Input: part model. Units: mm. Frame: model coordinates. Coordinates: 2 decimals unless noted, no trailing zeros. Loops run counter-clockwise (first coordinate to the right, second up) from the corner with the lowest first, then second, coordinate; pieces in that order, holes last. Notation, with made-up numbers: (0, 44.25) -> (16, 44.25) arc R18 cw to (16, 54.25) -> close; hole circle Ø3 at (-4, -6.75). An arc over 180 degrees is marked (long way). Answer as a JSON object with one key per item and string values.
from build123d import *

# Parameters (mm, degrees)
SKETCH1_W                  = 76.2
SKETCH1_H                  = 76.2
SKETCH1_R                  = 14.2875
SKETCH1_R_2                = 2.54
INITIAL_PLATE_DEPTH        = 6.35
MOUNTING_PATTERN_OUTLINE_R = 2.54
MOUNTING_PATTERN_DEPTH     = 6.35


# Read off the part's stored shape, not the designer's step: Mounting Pattern
with BuildPart() as part:
    # Sketch1 → Initial Plate (new body)
    with BuildSketch(Plane(origin=(0, 0, 0), x_dir=(1, 0, 0), z_dir=(0, 1, 0))):
        Rectangle(SKETCH1_W, SKETCH1_H)
        with Locations(Location((0, 0, 0), (0, 0, 270))):
            Circle(SKETCH1_R, mode=Mode.SUBTRACT)
        with Locations(Location((-25.4, 0, 0), (0, 0, 270))):
            Circle(SKETCH1_R_2, mode=Mode.SUBTRACT)
    extrude(amount=INITIAL_PLATE_DEPTH)

    # Mounting Pattern outline → Mounting Pattern (cut)
    with BuildSketch(Plane(origin=(0, 0, 0), x_dir=(1, 0, 0), z_dir=(0, 1, 0))):
        with Locations((0, 25.4)):
            Circle(MOUNTING_PATTERN_OUTLINE_R)
        with Locations((25.4, 0)):
            Circle(MOUNTING_PATTERN_OUTLINE_R)
        with Locations((0, -25.4)):
            Circle(MOUNTING_PATTERN_OUTLINE_R)
    extrude(amount=MOUNTING_PATTERN_DEPTH, mode=Mode.SUBTRACT)


solid = part.part
1. Section query A-A (x = 25.4). Return loops of the section in (y, z).
Reply:
{"outline": "(0, -38.1) -> (6.35, -38.1) -> (6.35, -2.54) -> (0, -2.54) -> close; (0, 2.54) -> (6.35, 2.54) -> (6.35, 38.1) -> (0, 38.1) -> close"}
2. Section query C-C (y = 5). Return loops of the section in (x, z) (1 decimal), plus the area to 3 significant figures.
Reply:
{"outline": "(-38.1, -38.1) -> (38.1, -38.1) -> (38.1, 38.1) -> (-38.1, 38.1) -> close; hole circle Ø5.1 at (-25.4, 0); hole circle Ø28.6 at (0, 0); hole circle Ø5.1 at (0, -25.4); hole circle Ø5.1 at (0, 25.4); hole circle Ø5.1 at (25.4, 0)", "area": "5,080 mm2"}
3. Mould query, pull axis Z, two halves, no side actions, for faces 1 (the face through (16, 0, -1)), 2 (the face through (-27.653, 3.131, 1.172)), 3 (the face through (-1, 3, 38.1)). Classes: pulls with the +Z half, pulls with the -Z half, needs draft (parallel to the pull), parting line crosses it, or undercut.
Reply:
{"face 1": "needs draft", "face 2": "undercut", "face 3": "pulls with the +Z half"}
4. Section query B-B (z = 25.4). Return loops of the section in (x, y).
Reply:
{"outline": "(-38.1, 0) -> (-2.54, 0) -> (-2.54, 6.35) -> (-38.1, 6.35) -> close; (2.54, 0) -> (38.1, 0) -> (38.1, 6.35) -> (2.54, 6.35) -> close"}
5. Section query D-D (z = 0). Return loops of the section in (x, y), plus the area to 3 significant figures.
Reply:
{"outline": "(-38.1, 0) -> (-27.94, 0) -> (-27.94, 6.35) -> (-38.1, 6.35) -> close; (-22.86, 0) -> (-14.29, 0) -> (-14.29, 6.35) -> (-22.86, 6.35) -> close; (14.29, 0) -> (22.86, 0) -> (22.86, 6.35) -> (14.29, 6.35) -> close; (27.94, 0) -> (38.1, 0) -> (38.1, 6.35) -> (27.94, 6.35) -> close", "area": "238 mm2"}
6. Line query: line 1 along X through (y, z) = (1.75, 0); line 2 along Z through (x, y) = (2, 3); line 3 along Z through (x, y) = (25.4, 4.25). Output: solid intervals per line, ascending.
Reply:
{"line 1": "x = -38.1 to -27.94, -22.86 to -14.29, 14.29 to 22.86, 27.94 to 38.1", "line 2": "z = -38.1 to -26.97, -23.83 to -14.15, 14.15 to 23.83, 26.97 to 38.1", "line 3": "z = -38.1 to -2.54, 2.54 to 38.1"}
